Geometry check sheet. Reference: the model listing, model coordinates, mm. Face numbers are marked on the shaded views. Coordinates: 2 decimals unless noted, no trailing zeros. Loops run counter-clockwise (first coordinate to the right, second up) from the corner with the lowest first, then second, coordinate; pieces in that order, holes last. Notation, with made-up numbers: M 87.5,86.25 L 97.5,86.25 A13 ccw 97.5,94.25 Z; hole C 0.25,5.5 d9. An arc over 180 degrees is marked long. Use CSV: the item, a comma, the result in double quotes.
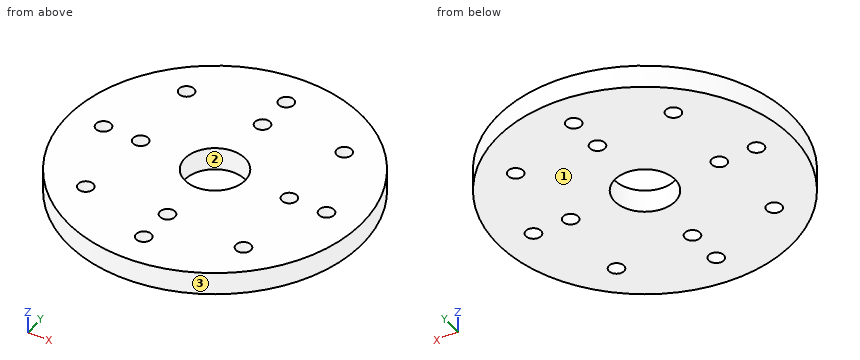
```python
from build123d import *

# Parameters (mm, degrees)
CROQUIS1_R              = 19.5
SALIENTE_EXTRUIR1_DEPTH = 3
CROQUIS2_R              = 1
CORTAR_EXTRUIR1_DEPTH   = 3
CROQUIS3_R              = 4
CORTAR_EXTRUIR2_DEPTH   = 3


with BuildPart() as part:
    # Croquis1 → Saliente-Extruir1 (new body)
    with BuildSketch(Plane.XY):
        Circle(CROQUIS1_R)
    extrude(amount=SALIENTE_EXTRUIR1_DEPTH)

    # Croquis2 → Cortar-Extruir1 (cut)
    with BuildSketch(Plane.XY.offset(3)):
        with Locations((0, 10)):
            Circle(CROQUIS2_R)
        with Locations((10, 0)):
            Circle(CROQUIS2_R)
        with Locations((0, -10)):
            Circle(CROQUIS2_R)
        with Locations((-10, 0)):
            Circle(CROQUIS2_R)
        with Locations((0, 15)):
            Circle(CROQUIS2_R)
        with Locations((10.606601718, 10.606601718)):
            Circle(CROQUIS2_R)
        with Locations((15, 0)):
            Circle(CROQUIS2_R)
        with Locations((10.606601718, -10.606601718)):
            Circle(CROQUIS2_R)
        with Locations((0, -15)):
            Circle(CROQUIS2_R)
        with Locations((-10.606601718, -10.606601718)):
            Circle(CROQUIS2_R)
        with Locations((-15, 0)):
            Circle(CROQUIS2_R)
        with Locations((-10.606601718, 10.606601718)):
            Circle(CROQUIS2_R)
    extrude(amount=-CORTAR_EXTRUIR1_DEPTH, mode=Mode.SUBTRACT)

    # Croquis3 → Cortar-Extruir2 (cut)
    with BuildSketch(Plane.XY.offset(3)):
        Circle(CROQUIS3_R)
    extrude(amount=-CORTAR_EXTRUIR2_DEPTH, mode=Mode.SUBTRACT)


solid = part.part
```
1. Gauge pin test, flat ends, axial feed: P1, Ø2.5, axis at x = 10.61, y = -10.61, coming from the +Z side; P2, Ø1.5, axis at y = -9.5, z = 2, coming from the +X side; P3, Ø1, axis at x = -1, z = 1.5, coming from the -Y side; P4, Ø1, axis at y = -10.5, z = 0.5, coming from the -X side. Record the tip position at first contact, or that the pin passes through.
The answers:
P1,"z = 3"
P2,"x = 17.43"
P3,"y = -19.49"
P4,"x = -16.74"
2. Thickness scan on line 1 (Y direction, x = 0, z = 1.75); line 2 (Y direction, x = -10, z = 2.05); line 3 (Y direction, x = 2.5, z = 1.6). Record the ranges inside material, lowest first. Write a range as [from, to].
The answers:
line 1,"[-19.5, -16], [-14, -11], [-9, -4], [4, 9], [11, 14], [16, 19.5]"
line 2,"[-16.74, -11.4], [-9.81, -1], [1, 9.81], [11.4, 16.74]"
line 3,"[-19.34, -3.12], [3.12, 19.34]"
3. Release check for a two-part mould opening along X. For the marked faces 1, 2 and 3 record: +X half, -X half, draft (parallel to the pull), parting line (faces both ways), or undercut.
The answers:
face 1,"draft"
face 2,"undercut"
face 3,"parting line"
4. Section check B-B, the plane y = 0. Record the cut outline in (x, z), plus the area to 3 significant figures.
The answers:
outline,"M -19.5,0 L -16,0 L -16,3 L -19.5,3 Z; M -14,0 L -11,0 L -11,3 L -14,3 Z; M -9,0 L -4,0 L -4,3 L -9,3 Z; M 4,0 L 9,0 L 9,3 L 4,3 Z; M 11,0 L 14,0 L 14,3 L 11,3 Z; M 16,0 L 19.5,0 L 19.5,3 L 16,3 Z"
area,"69.0 mm^2"
5. Section check A-A, the plane x = 2.5. Record the cut outline in (y, z), plus the area to 3 significant figures.
The answers:
outline,"M -19.34,0 L -3.12,0 L -3.12,3 L -19.34,3 Z; M 3.12,0 L 19.34,0 L 19.34,3 L 3.12,3 Z"
area,"97.3 mm^2"
6. Section check C-C, the plane z = 2.55. Count the separate pieces of the cut face and the enclosed holes in it, plus the area to 3 significant figures.
The answers:
separate pieces,"1"
enclosed holes,"13"
area,"1,110 mm^2"
7. Section check D-D, the plane y = -15.5. Record the cut outline in (x, z).
The answers:
outline,"M -11.83,0 L -0.87,0 L -0.87,3 L -11.83,3 Z; M 0.87,0 L 11.83,0 L 11.83,3 L 0.87,3 Z"
